Geometry: see drawing. Coordinates: mm, zero at the bounding-box minimum. Round coordinates to 2 decimals unless told otherwise and drop trailing zeros. Write each loop counter-clockwise with the first axis right and the second up, starting at its lowest first coordinate (ties: lowest second). Pieces come first, ordered by that corner, then holes. Notation, with made-up numbers: M -4,78 L 26,78 A25 ccw 26,97 Z; hole C 8.5,53 d6. An arc over 180 degrees is marked long. Use a Markdown table: item, result.
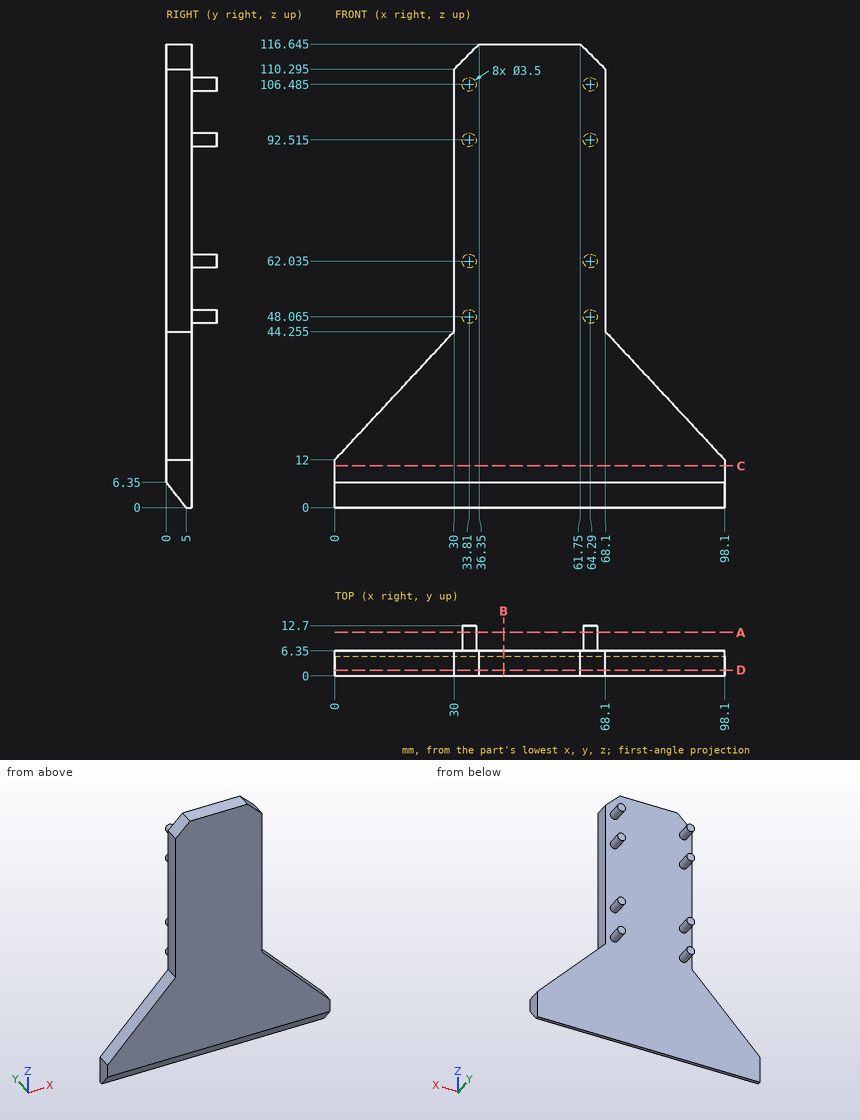
Q1. Section C-C on z = 10.5. Return loops of the section in (x, y), plus the area to 3 significant figures.
Results are:
| item | result |
|---|---|
| outline | M 0,0 L 98.1,0 L 98.1,6.35 L 0,6.35 Z |
| area | 623 mm^2 |
Q2. Section D-D on y = 1.5. Return loops of the section in (x, z) (3 decimals).
Results are:
| item | result |
|---|---|
| outline | M 0,4.445 L 98.1,4.445 L 98.1,12 L 68.1,44.255 L 68.1,110.295 L 61.75,116.645 L 36.35,116.645 L 30,110.295 L 30,44.255 L 0,12 Z |
Q3. First-contact query: pin 1 Ø3 at (y, z) = (3, 86) entering from -X; pin 2 Ø3 at (x, y) = (70.5, 2) entering from +Z; pin 3 Ø10 at (x, z) = (22.5, 18.5) entering from +Y. Flat tips, straight axial feed; report the tip coordinate or a pass-through.
Results are:
| item | result |
|---|---|
| pin 1 | x = 30 |
| pin 2 | z = 43.29 |
| pin 3 | y = 6.35 |
Q4. Line query: L1, parallel to Y at x = 55, z = 64; L2, parallel to X at y = 1.25, z = 45; L3, parallel to X at y = 7.75, z = 105.5. Output: solid intervals per line, ascending.
Results are:
| item | result |
|---|---|
| L1 | 0 to 6.35 |
| L2 | 30 to 68.1 |
| L3 | 32.36 to 35.26, 62.84 to 65.74 |
Q5. Section A-A on y = 11. Return loops of the section in (x, z) (3 decimals), plus the area to 3 significant figures.
Results are:
| item | result |
|---|---|
| outline | C 33.81,48.065 d3.5; C 33.81,62.035 d3.5; C 33.81,92.515 d3.5; C 33.81,106.485 d3.5; C 64.29,48.065 d3.5; C 64.29,62.035 d3.5; C 64.29,92.515 d3.5; C 64.29,106.485 d3.5 |
| area | 77.0 mm^2 |
Q6. Section B-B on x = 42.5. Return loops of the section in (y, z) (3 decimals), plus the area to 3 significant figures.
Results are:
| item | result |
|---|---|
| outline | M 0,6.35 L 5,0 L 6.35,0 L 6.35,116.645 L 0,116.645 Z |
| area | 725 mm^2 |
